Check sheet for the modelled part. Datum: model origin and axes. Units: mm. Face numbers are marked on the shaded views. Give positions to 0.01 mm unless a question says otherwise; leave off trailing zeros. Loops run counter-clockwise (first coordinate to the right, second up) from the corner with the lowest first, then second, coordinate; pieces in that order, holes last. Notation, with made-up numbers: (70, 27.25) - (119, 27.25) arc R26 ccw to (119, 47.25) - close; hole circle Ø9 at (45, 12.25). An arc over 180 degrees is marked (long way). Use CSV: the item, a comma, the result in double quotes.
Autodesk Inventor part; units mm, degrees
ref_plane "YZ Plane" through (0, 0, 0) normal (1, 0, 0) x (0, 1, 0)
ref_plane "XZ Plane" through (0, 0, 0) normal (0, 1, 0) x (-1, 0, 0)
ref_plane "XY Plane" through (0, 0, 0) normal (0, 0, 1) x (1, 0, 0)
sketch "スケッチ1" plane through (0, 0, 0) normal (0, 0, 1) x (1, 0, 0)
  circle A0 centre (0, 0) radius 2.5
  dimension "d0" = 5
extrude "押し出し1" add sketch "スケッチ1" along normal blind 5
sketch "スケッチ2" plane through (0, 0, 0) normal (1, 0, 0) x (0, 1, 0)
  line L0 (2.5, 5) -> (-2.5, 5)
  line L1 (2.5, 0) -> (-2.5, 0)
  circle A0 centre (0, 9) radius 2
  circle A1 centre (0, 9) radius 4
  line L2 (2.5, 5) -> (-2.5, 5)
  point P0 (0, 0)
  dimension "d3" = 4
  dimension "d4" = 8
sketch "スケッチ3" plane through (0, 0, 5) normal (0, 0, 1) x (1, 0, 0)
  circle A0 centre (0, 0) radius 2.5
extrude "押し出し2" add sketch "スケッチ3" along normal blind 1
extrude "押し出し3" add sketch "スケッチ2" along normal mid plane 3
properties part number "尻" material "ABS プラスチック"
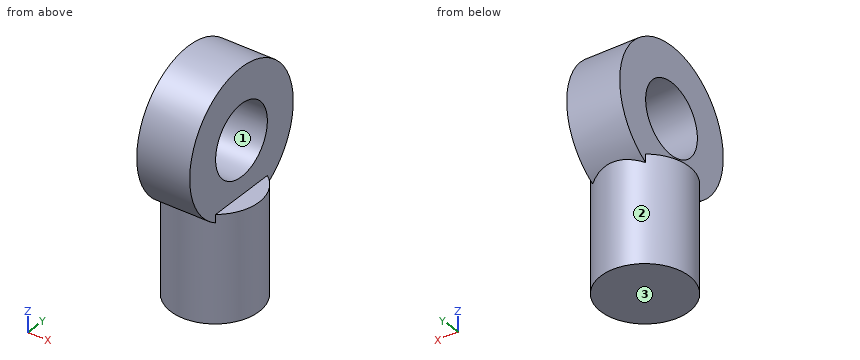
1. Sectioned sample at B-B, the plane y = 0.75. Record the boundary of the cut face in (x, z).
Completed:
outline,"(-2.38, 0) - (2.38, 0) - (2.38, 6) - (1.5, 6) - (1.5, 7.15) - (-1.5, 7.15) - (-1.5, 6) - (-2.38, 6) - close; (-1.5, 10.85) - (1.5, 10.85) - (1.5, 12.93) - (-1.5, 12.93) - close"
2. Scan lines: line 1 along Z through (x, y) = (0.7, 0); line 2 along Z through (x, y) = (-1.4, -0.75); line 3 along X through (y, z) = (3.25, 7.5). Record each from-to range of solid material in increasing order.
Completed:
line 1,"z = 0 to 7, 11 to 13"
line 2,"z = 0 to 7.15, 10.85 to 12.93"
line 3,"x = -1.5 to 1.5"
3. Go/stop test with flat-tipped pins: pin 1 Ø1.1 at (x, y) = (-2, 0.5) entering from +Z; pin 2 Ø1.1 at (x, y) = (2, 1) entering from +Z (3 decimals); pin 3 Ø3 at (y, z) = (-2, 5.5) entering from -X. Record where each tip stops, or that it passes through.
Completed:
pin 1,"stops at z = 12.99"
pin 2,"stops at z = 12.925"
pin 3,"stops at x = -2.45"
4. Sectioned sample at C-C, the plane x = 0. Record the boundary of the cut face in (y, z).
Completed:
outline,"(-2.5, 0) - (2.5, 0) - (2.5, 5.88) arc R4 ccw (long way) to (-2.5, 5.88) - close; hole circle Ø4 at (0, 9)"
5. Sectioned sample at D-D, the plane z = 7.25. Record the boundary of the cut face in (x, y).
Completed:
outline,"(-1.5, -3.6) - (1.5, -3.6) - (1.5, -0.97) - (-1.5, -0.97) - close; (-1.5, 0.97) - (1.5, 0.97) - (1.5, 3.6) - (-1.5, 3.6) - close"
6. Release check for a two-part mould opening along Z. For the marked faces 1, 2 and 3 record: released by +Z, released by -Z, zero draft, split by the parting line, or undercut.
Completed:
face 1,"undercut"
face 2,"zero draft"
face 3,"released by -Z"
7. Sectioned sample at A-A, the plane z = 9. Record the boundary of the cut face in (x, y).
Completed:
outline,"(-1.5, -4) - (1.5, -4) - (1.5, -2) - (-1.5, -2) - close; (-1.5, 2) - (1.5, 2) - (1.5, 4) - (-1.5, 4) - close"
